from build123d import *

# Parameters (mm, degrees)
SKETCH1_R           = 19.05
BOSS_EXTRUDE1_DEPTH = 1.143
SKETCH2_R           = 22.225
BOSS_EXTRUDE2_DEPTH = 1.27
SKETCH3_R           = 3.556
CUT_EXTRUDE1_DEPTH  = 5.826
SKETCH4_R           = 0.5715
CUT_EXTRUDE3_DEPTH  = 5.826
SKETCH5_R           = 0.5715
CUT_EXTRUDE4_DEPTH  = 5.826
CUT_EXTRUDE5_DEPTH  = 1.778
SKETCH10_R          = 0.5715
CUT_EXTRUDE6_DEPTH  = 5.826
SKETCH11_R          = 3.81
CUT_EXTRUDE7_DEPTH  = 5.826


with BuildPart() as part:
    # Sketch1 → Boss-Extrude1 (new body, symmetric)
    with BuildSketch(Plane.XY):
        Circle(SKETCH1_R)
    extrude(amount=BOSS_EXTRUDE1_DEPTH, both=True)

    # Sketch2 → Boss-Extrude2 (add)
    with BuildSketch(Plane.XY.offset(1.143)):
        Circle(SKETCH2_R)
    boss_extrude2 = extrude(amount=BOSS_EXTRUDE2_DEPTH)

    # Mirror1: Boss-Extrude2 across plane
    add(boss_extrude2.mirror(Plane.XY))

    # Sketch3 → Cut-Extrude1 (cut, through all)
    with BuildSketch(Plane(origin=(0, 0, -2.413), x_dir=(-1, 0, 0), z_dir=(0, 0, -1))):
        Circle(SKETCH3_R)
    extrude(amount=-CUT_EXTRUDE1_DEPTH, mode=Mode.SUBTRACT)

    # Sketch4 → Cut-Extrude3 (cut, through all)
    with BuildSketch(Plane(origin=(0, 0, -2.413), x_dir=(-1, 0, 0), z_dir=(0, 0, -1))):
        with Locations((12.8905, 0)):
            Circle(SKETCH4_R)
        with Locations((6.5405, 0)):
            Circle(SKETCH4_R)
        with Locations((-12.8905, 0)):
            Circle(SKETCH4_R)
        with Locations((-6.5405, 0)):
            Circle(SKETCH4_R)
    extrude(amount=-CUT_EXTRUDE3_DEPTH, mode=Mode.SUBTRACT)

    # Sketch5 → Cut-Extrude4 (cut, through all)
    with BuildSketch(Plane(origin=(0, 0, -2.413), x_dir=(-1, 0, 0), z_dir=(0, 0, -1))):
        with Locations((-18.542, 8.89)):
            Circle(SKETCH5_R)
    extrude(amount=-CUT_EXTRUDE4_DEPTH, mode=Mode.SUBTRACT)

    # Sketch7 → Cut-Extrude5 (cut)
    with BuildSketch(Plane(origin=(0, 0, -2.413), x_dir=(-1, 0, 0), z_dir=(0, 0, -1))):
        with BuildLine():
            Line((-1.9177, 3.6195), (-1.9177, 6.4262))
            ThreePointArc((-1.9177, 6.4262), (0, 8.3439), (1.9177, 6.4262))
            Line((1.9177, 6.4262), (1.9177, 2.921))
            Line((1.9177, 2.921), (14.672772863, 2.0955))
            ThreePointArc((14.672772863, 2.0955), (16.383, 0), (14.672772863, -2.0955))
            Line((14.672772863, -2.0955), (1.9177, -2.921))
            Line((1.9177, -2.921), (1.9177, -6.4262))
            ThreePointArc((1.9177, -6.4262), (0, -8.3439), (-1.9177, -6.4262))
            Line((-1.9177, -6.4262), (-1.9177, -3.6195))
            Line((-1.9177, -3.6195), (-16.902805323, -2.0955))
            ThreePointArc((-16.902805323, -2.0955), (-18.796, 0), (-16.902805323, 2.0955))
            Line((-16.902805323, 2.0955), (-1.9177, 3.6195))
        make_face()
    extrude(amount=-CUT_EXTRUDE5_DEPTH, mode=Mode.SUBTRACT)

    # Sketch10 → Cut-Extrude6 (cut, through all)
    with BuildSketch(Plane(origin=(0, 0, -2.413), x_dir=(-1, 0, 0), z_dir=(0, 0, -1))):
        with Locations((0, -6.223)):
            Circle(SKETCH10_R)
        with Locations((0, 6.223)):
            Circle(SKETCH10_R)
    extrude(amount=-CUT_EXTRUDE6_DEPTH, mode=Mode.SUBTRACT)

    # Sketch11 → Cut-Extrude7 (cut, through all)
    with BuildSketch(Plane(origin=(0, 0, -2.413), x_dir=(-1, 0, 0), z_dir=(0, 0, -1))):
        Circle(SKETCH11_R)
    extrude(amount=-CUT_EXTRUDE7_DEPTH, mode=Mode.SUBTRACT)


solid = part.part
CAD build for the part. Positions are in the model's coordinates, mm. A direction names the side the tool comes from. Round coordinates to 2 decimals unless told otherwise and drop trailing zeros. Loops run counter-clockwise (first coordinate to the right, second up) from the corner with the lowest first, then second, coordinate; pieces in that order, holes last.
(1) Cut at A-A (x = 0). State how many separate pieces and enclosed holes the cut face has, plus the area to 3 significant figures.
(2) Which spindle directions (+Z, -Z, +X, -X, +Y, -Y) get a long thin tool onto all of the face, cutting with end or side? Do faces 5 (the flat face through (-1.918, 5, -2)), 6 (the cylindrical face through (19.113, 8.915, 1.769)), 7 (the cylindrical face through (-15.12, -11.59, 0.02)). Say none if no direction does.
(3) Two-plate mould, pull along Y, no slides. Class faces 1 (the flat face through (5, -5, -2.413)), 2 (the flat face through (-10, 0, -0.635)), 3 (the cylindrical face through (21.199, 6.676, 1.769)), 4 (the cylindrical face through (18.796, -0.043, -1.536)): +Y half, -Y half, draft (parallel to the pull), parting line (faces both ways), or undercut.
(4) Cut at D-D (y = -7.5). Give the cut face in (x, z) (1 decimal), plus the area to 3 significant figures.
(5) Cut at C-C (y = -1.5). Give the cut face in (x, z) (3 decimals), plus the area to 3 significant figures.
(6) Wall check: line 1 along Y through (x, z) = (0, -0.15); line 2 along Z through (x, y) = (19, 7.5); line 3 along Z through (x, y) = (-1, -5) (3 decimals). Give the ranges that are in metal, low to high.
(7) Drop flat-ended pins along their axis: pin 1 (1.3 mm diameter, centred on x = 0, y = -6.223, fed in from -Z) (3 decimals); pin 2 (0.5 mm diameter, centred on y = -5.5, z = -2, fed in from -X); pin 3 (0.5 mm diameter, centred on y = -4.5, z = -1.5, fed in from +X). Give the stop position or say it passes through.
Findings below:
1. separate pieces: 4
1. enclosed holes: 0
1. area: 140 mm2
2. face 5: -Z
2. face 6: +Z, -Z
2. face 7: none
3. face 1: draft
3. face 2: undercut
3. face 3: parting line
3. face 4: undercut
4. outline: (-20.9, -2.4) - (-1.6, -2.4) - (-1.6, -0.6) - (1.6, -0.6) - (1.6, -2.4) - (20.9, -2.4) - (20.9, -1.1) - (17.5, -1.1) - (17.5, 1.1) - (20.9, 1.1) - (20.9, 2.4) - (-20.9, 2.4) - (-20.9, 1.1) - (-17.5, 1.1) - (-17.5, -1.1) - (-20.9, -1.1) - close
4. area: 181 mm2
5. outline: (-22.174, -2.413) - (-15.769, -2.413) - (-15.769, -0.635) - (-3.502, -0.635) - (-3.502, 2.413) - (-22.174, 2.413) - (-22.174, 1.143) - (-18.991, 1.143) - (-18.991, -1.143) - (-22.174, -1.143) - close; (3.502, -0.635) - (18.168, -0.635) - (18.168, -2.413) - (22.174, -2.413) - (22.174, -1.143) - (18.991, -1.143) - (18.991, 1.143) - (22.174, 1.143) - (22.174, 2.413) - (3.502, 2.413) - close
5. area: 118 mm2
6. line 1: y = -19.05 to -6.79, -5.65 to -3.81, 3.81 to 5.65, 6.79 to 19.05
6. line 2: z = -2.41 to -1.14, 1.14 to 2.41
6. line 3: z = -0.635 to 2.413
7. pin 1: stops at z = -0.635
7. pin 2: stops at x = -21.6
7. pin 3: stops at x = 21.81
